Could you check a few things on this drawing? It's one solid part, dimensions in mm from its lowest x, y, z. A direction names the side the tool comes from. Round coordinates to 2 decimals unless told otherwise and drop trailing zeros. Write each loop counter-clockwise with the first axis right and the second up, starting at its lowest first coordinate (ties: lowest second). Pieces come first, ordered by that corner, then holes. Notation, with made-up numbers: (17.5, 3) - (42.5, 3) arc R8 ccw to (42.5, 17) - close; hole circle Ø10 at (17.5, -3). An arc over 180 degrees is marked (long way). Use one line per item in the form item = value. Start each with the question number.
1. I want a section at A-A, the plane x = 10.5. List the corners of the cut face in (y, z) for me (1 decimal).
2. Which directions (+Z, -Z, +X, -X, +Y, -Y) give clear straight access to the entire face, cutting with the end or side of a thin tool? Please do the marked faces 1 and 2.
3. Will these pins go through, and if not, where does the flat tip stop? pin 1 (8 mm diameter, centred on y = 5, z = 4, fed in from -X); pin 2 (6 mm diameter, centred on y = 22.5, z = 10, fed in from -X); pin 3 (1 mm diameter, centred on x = 15, z = 19, fed in from +Y); pin 4 (10 mm diameter, centred on y = 5.5, z = 13, fed in from +X).
4. We'd pull the mould along Y, two halves only. Please class the marked faces 3, 4 and 5: +Y half, -Y half, draft (parallel to the pull), parting line (faces both ways), or undercut.
5. If I drill on line 1 along Z through (x, y) = (4.5, 23); line 2 along X through (y, z) = (8.75, 18.5) (1 decimal); line 3 along Y through (x, z) = (21.5, 19.75) (1 decimal), over which ranges is the centre line in solid material (lowest first)?
6. I want a section at D-D, the plane z = 23. List the corners of the cut face in (x, y) for me.
7. I want a section at C-C, the plane y = 19. List the corners of the cut face in (x, z) for me, plus the area to 3 significant figures.
8. I want a section at B-B, the plane z = 15.75. List the corners of the cut face in (x, y) for me.
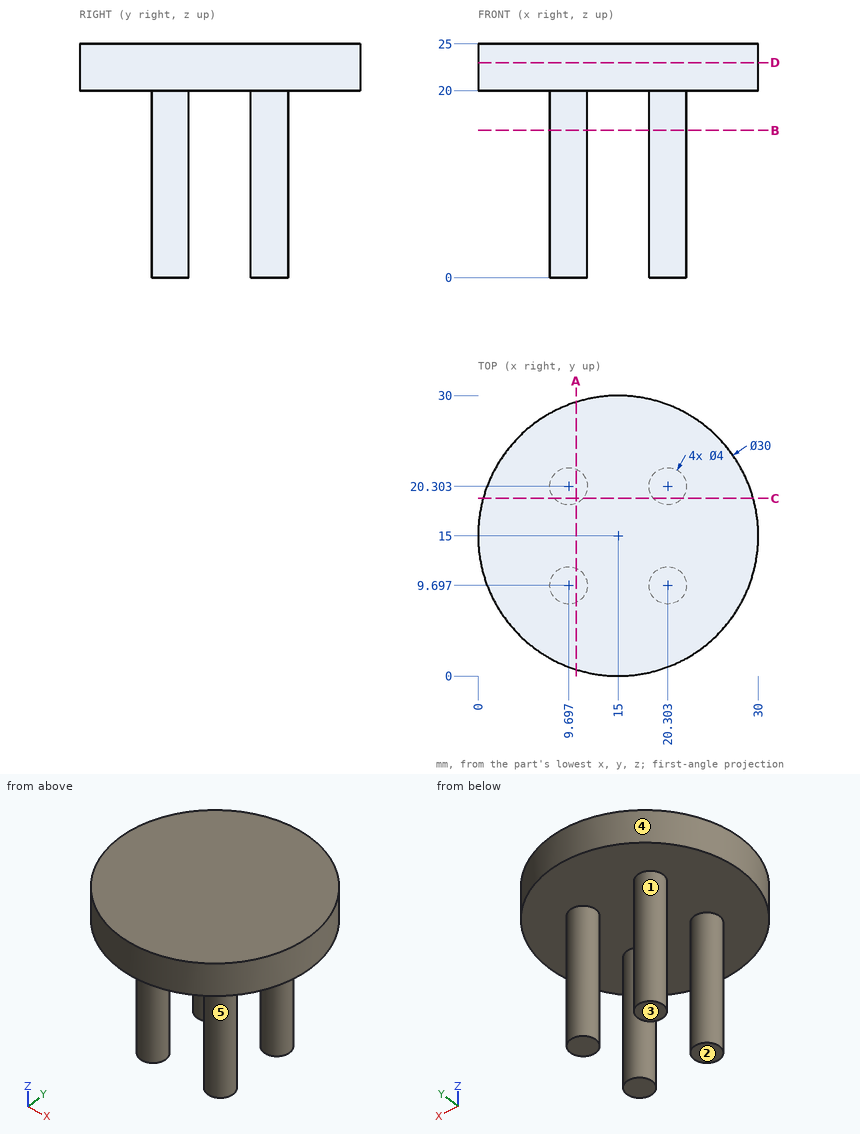
Model answer:
q1.outline = (0.7, 20) - (7.9, 20) - (7.9, 0) - (11.5, 0) - (11.5, 20) - (18.5, 20) - (18.5, 0) - (22.1, 0) - (22.1, 20) - (29.3, 20) - (29.3, 25) - (0.7, 25) - close
q2.face_1 = -Z
q2.face_2 = -Z, +X, -X, +Y, -Y
q3.pin_1 = 7.82
q3.pin_2 = 7.7
q3.pin_3 = through
q3.pin_4 = 22.3
q4.face_3 = draft
q4.face_4 = parting line
q4.face_5 = undercut
q5.line_1 = 20 to 25
q5.line_2 = 7.9 to 11.5, 18.5 to 22.1
q5.line_3 = 8.1 to 11.3, 18.7 to 21.9
q6.outline = circle Ø30 at (15, 15)
q7.outline = (0.54, 20) - (8.18, 20) - (8.18, 0) - (11.21, 0) - (11.21, 20) - (18.79, 20) - (18.79, 0) - (21.82, 0) - (21.82, 20) - (29.46, 20) - (29.46, 25) - (0.54, 25) - close
q7.area = 266 mm2
q8.outline = circle Ø4 at (9.7, 9.7); circle Ø4 at (9.7, 20.3); circle Ø4 at (20.3, 9.7); circle Ø4 at (20.3, 20.3)
